```python
from build123d import *

# Parameters (mm, degrees)
SKETCH_1_W          = 152
SKETCH_1_H          = 84
EXTRUDE_1_DEPTH     = 1.8
SKETCH_3_R          = 1.64
SKETCH_3_R_2        = 1.462072503
EXTRUDE_2_DEPTH     = 28
SKETCH_3_2_R        = 1.64
SKETCH_3_2_R_2      = 1.462072503
EXTRUDE_3_DEPTH     = 4.5
EXTRUDE_START       = -24
EXTRUDE_4_OUTLINE_R = 2
EXTRUDE_4_DEPTH     = 2
SKETCH_10_W         = 1.8
SKETCH_10_H         = 84
EXTRUDE_6_DEPTH     = 30


# Read off the part's stored shape, not the designer's step: the extrude step
with BuildPart() as part:
    # Sketch 1 → Extrude 1 (new body)
    with BuildSketch(Plane(origin=(0, 0, 0), x_dir=(1, 0, 0), z_dir=(0, 1, 0))):
        with Locations((76, 42)):
            Rectangle(SKETCH_1_W, SKETCH_1_H)
    extrude(amount=EXTRUDE_1_DEPTH)

    # Sketch 3 → Extrude 2 (add)
    with BuildSketch(Plane(origin=(0, 1.8, 0), x_dir=(1, 0, 0), z_dir=(0, 1, 0))):
        with Locations(Location((143.5, 8.5, 0), (0, 0, 270))):
            Circle(SKETCH_3_R)
        with Locations(Location((143.5, 64.5, 0), (0, 0, 270))):
            Circle(SKETCH_3_R_2)
        with BuildLine():
            Line((8.15, 10.14), (9.85, 10.14))
            ThreePointArc((9.85, 10.14), (11.49, 8.5), (9.85, 6.86))
            Line((9.85, 6.86), (8.15, 6.86))
            ThreePointArc((8.15, 6.86), (6.51, 8.5), (8.15, 10.14))
        make_face()
        with BuildLine():
            Line((8.15, 73.84), (9.85, 73.84))
            ThreePointArc((9.85, 73.84), (11.49, 75.48), (9.85, 77.12))
            Line((9.85, 77.12), (8.15, 77.12))
            ThreePointArc((8.15, 77.12), (6.51, 75.48), (8.15, 73.84))
        make_face()
    extrude(amount=EXTRUDE_2_DEPTH)

    # Sketch 3_2 → Extrude 3 (add)
    with BuildSketch(Plane(origin=(0, 1.8, 0), x_dir=(1, 0, 0), z_dir=(0, 1, 0))):
        with Locations(Location((143.5, 8.5, 0), (0, 0, 270))):
            Circle(SKETCH_3_2_R)
        with Locations(Location((143.5, 64.5, 0), (0, 0, 270))):
            Circle(SKETCH_3_2_R_2)
        with BuildLine():
            Line((8.15, 10.14), (9.85, 10.14))
            ThreePointArc((9.85, 10.14), (11.49, 8.5), (9.85, 6.86))
            Line((9.85, 6.86), (8.15, 6.86))
            ThreePointArc((8.15, 6.86), (6.51, 8.5), (8.15, 10.14))
        make_face()
        with BuildLine():
            Line((8.15, 73.84), (9.85, 73.84))
            ThreePointArc((9.85, 73.84), (11.49, 75.48), (9.85, 77.12))
            Line((9.85, 77.12), (8.15, 77.12))
            ThreePointArc((8.15, 77.12), (6.51, 75.48), (8.15, 73.84))
        make_face()
    extrude(amount=EXTRUDE_3_DEPTH)

    # Extrude 4 outline → Extrude 4 (add)
    with BuildSketch(Plane(origin=(0, 29.8, 0), x_dir=(1, 0, 0), z_dir=(0, 1, 0)).offset(EXTRUDE_START)):
        with BuildLine():
            ThreePointArc((7.952208314, 10.5), (5.952208314, 8.5), (7.952208314, 6.5))
            Line((7.952208314, 6.5), (10.047791686, 6.5))
            ThreePointArc((10.047791686, 6.5), (12.047791686, 8.5), (10.047791686, 10.5))
            Line((10.047791686, 10.5), (7.952208314, 10.5))
        make_face()
        with BuildLine():
            ThreePointArc((7.952208314, 77.5), (5.952208314, 75.5), (7.952208314, 73.5))
            Line((7.952208314, 73.5), (10.047791686, 73.5))
            ThreePointArc((10.047791686, 73.5), (12.047791686, 75.5), (10.047791686, 77.5))
            Line((10.047791686, 77.5), (7.952208314, 77.5))
        make_face()
        with Locations((143.5, 64.5)):
            Circle(EXTRUDE_4_OUTLINE_R)
        with Locations((143.5, 8.5)):
            Circle(EXTRUDE_4_OUTLINE_R)
    extrude(amount=EXTRUDE_4_DEPTH)

    # Sketch 10 → Extrude 6 (add)
    with BuildSketch(Plane(origin=(0, 1.8, 0), x_dir=(1, 0, 0), z_dir=(0, 1, 0))):
        with Locations((0.9, 42)):
            Rectangle(SKETCH_10_W, SKETCH_10_H)
        with Locations((151.1, 42)):
            Rectangle(SKETCH_10_W, SKETCH_10_H)
    extrude(amount=EXTRUDE_6_DEPTH)


solid = part.part
```
The listing builds one solid part. Answer for the finished solid, in the listing's coordinates (mm). A direction names the side the tool comes from. Give positions to 0.01 mm unless a question says otherwise; leave off trailing zeros. Write each loop counter-clockwise with the first axis right and the second up, starting at its lowest first coordinate (ties: lowest second). Pieces come first, ordered by that corner, then holes. Notation, with made-up numbers: (-16, 64) -> (-2, 64) arc R11 ccw to (-2, 85) -> close; hole circle Ø6 at (14.25, -40). An arc over 180 degrees is marked (long way). Write item = value, one per line. Start each with the question number.
1) Which of the six approach directions +Z, -Z, +X, -X, +Y, -Y give full straight-line access (tool end or side, diameter ignored) to faces 1 (the face through (11.49, 3.77, -8.54)), 2 (the face through (1.8, 17, -41)), 3 (the face through (141.502, 6.786, -8.588))?
2) The part is cut by section B-B, the plane z = -64.5. Determine the outline of the cut face in (x, y), and give its area (3 significant figures).
3) Determine the mould class of faces 4 (the face through (76, 1, 0)), 5 (the face through (9, 29.8, -76)), 6 (the face through (0, 16, -41)), 7 (the face through (9, 5.8, -77.3)) for opening direction X: +X half, -X half, draft (parallel to the pull), parting line (faces both ways), or undercut.
4) The part is cut by section A-A, the plane y = 18.5. Determine the outline of the cut face in (x, z).
5) The part is cut by section D-D, the plane z = -75.5. Determine the outline of the cut face in (x, y), and give its area (3 significant figures).
6) The part is cut by section C-C, the plane x = 143.5. Determine the outline of the cut face in (y, z).
7) Straight lines are drawn through the part: line 1 along X through (y, z) = (5, -24); line 2 along X through (y, z) = (10.5, -74.5) (3 decimals); line 3 along Y through (x, z) = (28, -70). For each, find the intervals that lie inside material, in ascending order.
8) Each of these flat-tipped pins is pushed along its axis until it touches: pin 1 (0.8 mm diameter, centred on x = 9.5, y = 3, fed in from -Z); pin 2 (1.5 mm diameter, centred on y = 16, z = -56.5, fed in from -X); pin 3 (3 mm diameter, centred on x = 132.5, z = -22, fed in from +Y); pin 4 (1.6 mm diameter, centred on x = 9, y = 7, fed in from +Z). Where does it stop, or does it pass through?
Solutions:
q1.face_1 = none
q1.face_2 = +Z, -Z, +Y
q1.face_3 = +Y
q2.outline = (0, 0) -> (152, 0) -> (152, 31.8) -> (150.2, 31.8) -> (150.2, 1.8) -> (144.96, 1.8) -> (144.96, 5.8) -> (145.5, 5.8) -> (145.5, 7.8) -> (144.96, 7.8) -> (144.96, 29.8) -> (142.04, 29.8) -> (142.04, 7.8) -> (141.5, 7.8) -> (141.5, 5.8) -> (142.04, 5.8) -> (142.04, 1.8) -> (1.8, 1.8) -> (1.8, 31.8) -> (0, 31.8) -> close
q2.area = 466 mm²
q3.face_4 = draft
q3.face_5 = undercut
q3.face_6 = -X half
q3.face_7 = undercut
q4.outline = (0, -84) -> (1.8, -84) -> (1.8, 0) -> (0, 0) -> close; (8.15, -77.12) -> (9.85, -77.12) arc R1.64 ccw to (9.85, -73.84) -> (8.15, -73.84) arc R1.64 ccw to start; (8.15, -10.14) -> (9.85, -10.14) arc R1.64 ccw to (9.85, -6.86) -> (8.15, -6.86) arc R1.64 ccw to start; circle Ø3.28 at (143.5, -8.5); circle Ø2.92 at (143.5, -64.5); (150.2, -84) -> (152, -84) -> (152, 0) -> (150.2, 0) -> close
q5.outline = (0, 0) -> (152, 0) -> (152, 31.8) -> (150.2, 31.8) -> (150.2, 1.8) -> (11.49, 1.8) -> (11.49, 5.8) -> (12.05, 5.8) -> (12.05, 7.8) -> (11.49, 7.8) -> (11.49, 29.8) -> (6.51, 29.8) -> (6.51, 7.8) -> (5.95, 7.8) -> (5.95, 5.8) -> (6.51, 5.8) -> (6.51, 1.8) -> (1.8, 1.8) -> (1.8, 31.8) -> (0, 31.8) -> close
q5.area = 523 mm²
q6.outline = (0, -84) -> (1.8, -84) -> (1.8, -65.96) -> (5.8, -65.96) -> (5.8, -66.5) -> (7.8, -66.5) -> (7.8, -65.96) -> (29.8, -65.96) -> (29.8, -63.04) -> (7.8, -63.04) -> (7.8, -62.5) -> (5.8, -62.5) -> (5.8, -63.04) -> (1.8, -63.04) -> (1.8, -10.14) -> (5.8, -10.14) -> (5.8, -10.5) -> (7.8, -10.5) -> (7.8, -10.14) -> (29.8, -10.14) -> (29.8, -6.86) -> (7.8, -6.86) -> (7.8, -6.5) -> (5.8, -6.5) -> (5.8, -6.86) -> (1.8, -6.86) -> (1.8, 0) -> (0, 0) -> close
q7.line_1 = 0 to 1.8, 150.2 to 152
q7.line_2 = 0 to 1.8, 6.835 to 11.165, 150.2 to 152
q7.line_3 = 0 to 1.8
q8.pin_1 = -77.12
q8.pin_2 = 0
q8.pin_3 = 1.8
q8.pin_4 = -6.5
